Verification items for the finished model (mm, model axes). Give positions to 0.01 mm unless a question says otherwise; leave off trailing zeros. Order: outer loops, then holes, each group sorted by start corner. A loop starts at its lowest first (then second) coordinate and runs counter-clockwise, first axis right, second up. Notation, with made-up numbers: (61, 61) -> (86, 61) arc R37 cw to (86, 98) -> close; hole circle Ø9 at (-17, 17). An arc over 180 degrees is marked (long way). One line per question, with ' | ' between items. Start each with the question number.
Q1. Mould release check, pull along Z, two halves, no side actions. Record for faces 1 (the cylindrical face through (-11.5, 0, -27)), 2 (the flat face through (-29, 0, -30)), 3 (the flat face through (0, 0, -15)), 4 (the cylindrical face through (-52.44, -0.01, -15.54)): released by +Z, released by -Z, zero draft, split by the parting line, or undercut.
Q2. Material ranges on probe 1 along X at (y, z) = (0.5, -25); probe 2 along X at (y, z) = (0.15, -2.75); probe 3 along Z at (x, y) = (-9.5, 0), recorded low to high. Write a range as [from, to].
Q3. Section check B-B on z = -25. Record the cut outline in (x, y).
Q4. Section check A-A on x = -10. Record the cut outline in (y, z), plus the area to 3 significant figures.
Q5. Section check C-C on y = -0.05. Give the number of separate pieces and of enclosed holes in the cut face, plus the area to 3 significant figures.
from build123d import *

# Parameters (mm, degrees)
SKETCH2_W           = 57.4
SKETCH2_H           = 30
SKETCH2_R           = 2.5
BOSS_EXTRUDE1_DEPTH = 1.04


with BuildPart() as part:
    # Sketch2 → Boss-Extrude1 (new, symmetric)
    with BuildSketch(Plane(origin=(0, 0, 0), x_dir=(1, 0, 0), z_dir=(0, 1, 0))):
        with Locations((-28.7, 15)):
            Rectangle(SKETCH2_W, SKETCH2_H)
        with Locations(Location((-50, 25, 0), (0, 0, 270))):
            Circle(SKETCH2_R, mode=Mode.SUBTRACT)
        with Locations(Location((-50, 15, 0), (0, 0, 270))):
            Circle(SKETCH2_R, mode=Mode.SUBTRACT)
        with Locations(Location((-50, 5, 0), (0, 0, 270))):
            Circle(SKETCH2_R, mode=Mode.SUBTRACT)
        with Locations(Location((-30, 5, 0), (0, 0, 270))):
            Circle(SKETCH2_R, mode=Mode.SUBTRACT)
        with Locations(Location((-30, 15, 0), (0, 0, 270))):
            Circle(SKETCH2_R, mode=Mode.SUBTRACT)
        with Locations(Location((-30, 25, 0), (0, 0, 270))):
            Circle(SKETCH2_R, mode=Mode.SUBTRACT)
        with Locations(Location((-10, 5, 0), (0, 0, 270))):
            Circle(SKETCH2_R, mode=Mode.SUBTRACT)
        with Locations(Location((-10, 15, 0), (0, 0, 270))):
            Circle(SKETCH2_R, mode=Mode.SUBTRACT)
        with Locations(Location((-10, 25, 0), (0, 0, 270))):
            Circle(SKETCH2_R, mode=Mode.SUBTRACT)
    extrude(amount=BOSS_EXTRUDE1_DEPTH, both=True)


solid = part.part
Filled in:
1) face 1: undercut | face 2: released by -Z | face 3: zero draft | face 4: undercut
2) probe 1: [-57.4, -52.5], [-47.5, -32.5], [-27.5, -12.5], [-7.5, 0] | probe 2: [-57.4, -51.09], [-48.91, -31.09], [-28.91, -11.09], [-8.91, 0] | probe 3: [-30, -27.45], [-22.55, -17.45], [-12.55, -7.45], [-2.55, 0]
3) outline: (-57.4, -1.04) -> (-52.5, -1.04) -> (-52.5, 1.04) -> (-57.4, 1.04) -> close; (-47.5, -1.04) -> (-32.5, -1.04) -> (-32.5, 1.04) -> (-47.5, 1.04) -> close; (-27.5, -1.04) -> (-12.5, -1.04) -> (-12.5, 1.04) -> (-27.5, 1.04) -> close; (-7.5, -1.04) -> (0, -1.04) -> (0, 1.04) -> (-7.5, 1.04) -> close
4) outline: (-1.04, -30) -> (1.04, -30) -> (1.04, -27.5) -> (-1.04, -27.5) -> close; (-1.04, -22.5) -> (1.04, -22.5) -> (1.04, -17.5) -> (-1.04, -17.5) -> close; (-1.04, -12.5) -> (1.04, -12.5) -> (1.04, -7.5) -> (-1.04, -7.5) -> close; (-1.04, -2.5) -> (1.04, -2.5) -> (1.04, 0) -> (-1.04, 0) -> close | area: 31.2 mm²
5) separate pieces: 1 | enclosed holes: 9 | area: 1,550 mm²
